Can you work these out from the model? Positions are in its coordinate system, mm. A direction names the side the tool comes from. Round coordinates to 2 decimals unless told otherwise and drop trailing zeros. Loops run counter-clockwise (first coordinate to the right, second up) from the corner with the lowest first, then second, coordinate; pieces in that order, holes last. Notation, with made-up numbers: M -23,-18 L 34,-18 A21 ccw 34,11 Z; hole C 70.25,20 d9. An arc over 180 degrees is marked long. Return JSON: item names as keys, results as strings.
```python
from build123d import *

# Parameters (mm, degrees)
CUT_EXTRUDE1_START     = -2.025
CUT_EXTRUDE1_OUTLINE_W = 3.186396103
CUT_EXTRUDE1_OUTLINE_H = 1.6
CUT_EXTRUDE1_DEPTH     = 4.05
CUT_EXTRUDE1_START_2   = -1.575
CUT_EXTRUDE1_2_DEPTH   = 1.425
CUT_EXTRUDE1_START_3   = 0.15
CUT_EXTRUDE1_3_DEPTH   = 1.425
SKETCH2_W              = 0.3
SKETCH2_H              = 3.186396103
CUT_EXTRUDE2_DEPTH     = 0.3
CUT_EXTRUDE3_DEPTH     = 0.186396103
SKETCH4_W              = 3.45
SKETCH4_H              = 3
CUT_EXTRUDE4_DEPTH     = 1
BOSS_EXTRUDE1_DEPTH    = 6.2
SKETCH6_W              = 2.55
SKETCH6_H              = 0.3
BOSS_EXTRUDE2_DEPTH    = 0.75
SKETCH7_W              = 0.3
SKETCH7_H              = 0.6
BOSS_EXTRUDE3_DEPTH    = 0.3
SKETCH8_W              = 0.3
SKETCH8_H              = 0.6
BOSS_EXTRUDE4_DEPTH    = 0.3
SKETCH9_W              = 3.15
SKETCH9_H              = 0.3
BOSS_EXTRUDE5_DEPTH    = 1
SKETCH10_W             = 0.3
SKETCH10_H             = 6.05
BOSS_EXTRUDE6_DEPTH    = 0.45
SKETCH11_W             = 1.5
SKETCH11_H             = 0.3
BOSS_EXTRUDE7_DEPTH    = 1.05
SKETCH12_W             = 1.5
SKETCH12_H             = 0.3
BOSS_EXTRUDE8_DEPTH    = 1
SKETCH13_W             = 0.3
SKETCH13_H             = 6.05
BOSS_EXTRUDE9_DEPTH    = 0.45
DRAFT1_ANGLE           = 45
DRAFT2_ANGLE           = 45
FILLET1_R              = 0.15
FILLET2_R              = 0.45
FILLET3_R              = 0.6


with BuildPart() as part:
    # Cut-Extrude1: read off the stored shape, not the designer's step
    # Cut-Extrude1 outline → Cut-Extrude1 (new body)
    with BuildSketch(Plane.YZ.offset(CUT_EXTRUDE1_START)):
        with Locations((3.343198051, 0.8)):
            Rectangle(CUT_EXTRUDE1_OUTLINE_W, CUT_EXTRUDE1_OUTLINE_H)
    extrude(amount=CUT_EXTRUDE1_DEPTH)

    # Cut-Extrude1 2 outline → Cut-Extrude1 2 (add)
    with BuildSketch(Plane.YZ.offset(CUT_EXTRUDE1_START_2)):
        Polygon((4.936396103, 1.6), (4.936396103, 1.3), (5.73137085, 2.094974747), (4.812132034, 3.014213562), (4.812132034, 1.6), align=None)
        Polygon((1.189495749, 1.3), (1.75, 1.3), (1.75, 1.6), (1.15, 1.6), (-1.128726234, 0.989417146), (-2.09465206, 1.248236191), (-2.172297774, 0.958458443), (-1.128726234, 0.678834292), align=None)
    extrude(amount=CUT_EXTRUDE1_2_DEPTH)

    # Cut-Extrude1 3 outline → Cut-Extrude1 3 (add)
    with BuildSketch(Plane.YZ.offset(CUT_EXTRUDE1_START_3)):
        Polygon((4.936396103, 1.6), (4.936396103, 1.3), (5.73137085, 2.094974747), (4.812132034, 3.014213562), (4.812132034, 1.6), align=None)
        Polygon((1.189495749, 1.3), (1.75, 1.3), (1.75, 1.6), (1.15, 1.6), (-1.128726234, 0.989417146), (-2.09465206, 1.248236191), (-2.172297774, 0.958458443), (-1.128726234, 0.678834292), align=None)
    extrude(amount=CUT_EXTRUDE1_3_DEPTH)

    # Sketch2 → Cut-Extrude2 (cut)
    with BuildSketch(Plane.XY.offset(1.6)):
        with Locations((0, 3.343198051)):
            Rectangle(SKETCH2_W, SKETCH2_H)
    extrude(amount=-CUT_EXTRUDE2_DEPTH, mode=Mode.SUBTRACT)

    # Sketch3 → Cut-Extrude3 (cut)
    with BuildSketch(Plane(origin=(0, 4.936396103, 0), x_dir=(-1, 0, 0), z_dir=(0, 1, 0))):
        Polygon((-1.575, 1.3), (-1.575, 1.6), (-2.025, 1.6), (-2.025, 0), (2.025, 0), (2.025, 1.6), (1.575, 1.6), (1.575, 1.3), (0.15, 1.3), (-0.15, 1.3), align=None)
    extrude(amount=-CUT_EXTRUDE3_DEPTH, mode=Mode.SUBTRACT)

    # Sketch4 → Cut-Extrude4 (cut)
    with BuildSketch(Plane.XY.offset(1.3)):
        with Locations((0, 3.25)):
            Rectangle(SKETCH4_W, SKETCH4_H)
    extrude(amount=-CUT_EXTRUDE4_DEPTH, mode=Mode.SUBTRACT)

    # Sketch5 → Boss-Extrude1 (add)
    with BuildSketch(Plane.XZ.offset(-1.75)):
        Polygon((-1.725, 0.85), (-1.725, 0.3), (1.725, 0.3), (1.725, 0.85), (2.025, 0.85), (2.025, 0), (-2.025, 0), (-2.025, 0.85), align=None)
    extrude(amount=BOSS_EXTRUDE1_DEPTH)

    # Sketch6 → Boss-Extrude2 (add)
    with BuildSketch(Plane(origin=(0, 4.75, 0), x_dir=(-1, 0, 0), z_dir=(0, 1, 0))):
        with Locations((0, 0.15)):
            Rectangle(SKETCH6_W, SKETCH6_H)
    extrude(amount=BOSS_EXTRUDE2_DEPTH)

    # Sketch7 → Boss-Extrude3 (add)
    with BuildSketch(Plane.ZY.offset(1.275)):
        with Locations((0.15, 5.2)):
            Rectangle(SKETCH7_W, SKETCH7_H)
    extrude(amount=BOSS_EXTRUDE3_DEPTH)

    # Sketch8 → Boss-Extrude4 (add)
    with BuildSketch(Plane(origin=(1.275, 0, 0), x_dir=(0, 0, -1), z_dir=(1, 0, 0))):
        with Locations((-0.15, 5.2)):
            Rectangle(SKETCH8_W, SKETCH8_H)
    extrude(amount=BOSS_EXTRUDE4_DEPTH)

    # Sketch9 → Boss-Extrude5 (add)
    with BuildSketch(Plane(origin=(0, 0, 0), x_dir=(-1, 0, 0), z_dir=(0, 0, -1))):
        with Locations((0, 5.35)):
            Rectangle(SKETCH9_W, SKETCH9_H)
    extrude(amount=BOSS_EXTRUDE5_DEPTH)

    # Sketch10 → Boss-Extrude6 (add)
    with BuildSketch(Plane.XY.offset(0.85)):
        with Locations((-1.875, -1.425)):
            Rectangle(SKETCH10_W, SKETCH10_H)
    extrude(amount=BOSS_EXTRUDE6_DEPTH)

    # Sketch11 → Boss-Extrude7 (add)
    with BuildSketch(Plane.XZ.offset(4.45)):
        with Locations((0, 0.15)):
            Rectangle(SKETCH11_W, SKETCH11_H)
    extrude(amount=BOSS_EXTRUDE7_DEPTH)

    # Sketch12 → Boss-Extrude8 (add)
    with BuildSketch(Plane(origin=(0, 0, 0), x_dir=(-1, 0, 0), z_dir=(0, 0, -1))):
        with Locations((0, -5.35)):
            Rectangle(SKETCH12_W, SKETCH12_H)
    extrude(amount=BOSS_EXTRUDE8_DEPTH)

    # Sketch13 → Boss-Extrude9 (add)
    with BuildSketch(Plane.XY.offset(0.85)):
        with Locations((1.875, -1.425)):
            Rectangle(SKETCH13_W, SKETCH13_H)
    extrude(amount=BOSS_EXTRUDE9_DEPTH)

    # Draft1
    draft1_faces = [part.faces().sort_by_distance(p)[0] for p in [
        (0.8625, 4.812132034, 2.307106781),
    ]]
    draft(draft1_faces, Plane(origin=(0.960282071, 3.25, 1.6), x_dir=(1, 0, 0), z_dir=(0, 0, 1)), DRAFT1_ANGLE)

    # Draft2
    draft2_faces = [part.faces().sort_by_distance(p)[0] for p in [
        (-0.8625, 4.812132034, 2.307106781),
    ]]
    draft(draft2_faces, Plane(origin=(0.960282071, 3.25, 1.6), x_dir=(1, 0, 0), z_dir=(0, 0, 1)), DRAFT2_ANGLE)

    # Fillet1
    fillet1_edges = [part.edges().sort_by_distance(p)[0] for p in [
        (1.725, 3.25, 1.3),
        (0.8625, 1.189495749, 1.3),
        (0, -5.2, 0),
        (-0.8625, 4.812132034, 1.6),
        (0, 5.2, 0),
        (-1.725, 0.15, 0.3),
        (-0.8625, -1.128726234, 0.989417146),
        (-1.725, 3.25, 1.3),
        (0.8625, 4.812132034, 1.6),
        (0.8625, -1.128726234, 0.989417146),
        (-0.8625, 1.189495749, 1.3),
        (1.725, 0.15, 0.3),
    ]]
    fillet(fillet1_edges, radius=FILLET1_R)

    # Fillet2
    fillet2_edges = [part.edges().sort_by_distance(p)[0] for p in [
        (-2.025, 3.25, 1.6),
        (1.575, -2.133474917, 1.103347317),
        (0.15, -2.133474917, 1.103347317),
        (0.8625, -1.128726234, 0.678834292),
        (-0.8625, 4.936396103, 1.3),
        (0, 5.5, 0.3),
        (-0.8625, 1.15, 1.6),
        (2.025, 3.25, 1.6),
        (-0.15, -2.133474917, 1.103347317),
        (-1.575, -2.133474917, 1.103347317),
        (2.025, 0.15, 0),
        (-2.025, 0.15, 0),
        (0, -5.5, 0.3),
        (-0.8625, -1.128726234, 0.678834292),
        (0.8625, 4.936396103, 1.3),
        (0.8625, 1.15, 1.6),
    ]]
    fillet(fillet2_edges, radius=FILLET2_R)

    # Fillet3
    fillet3_edges = [part.edges().sort_by_distance(p)[0] for p in [
        (1.575, 5.625304833, 2.201040764),
        (1.875, -4.45, 1.3),
        (-1.875, -4.45, 1.3),
        (-0.75, -4.45, 0.15),
        (-1.575, 5.625304833, 2.201040764),
        (0.75, -4.45, 0.15),
    ]]
    fillet(fillet3_edges, radius=FILLET3_R)


solid = part.part
```
Q1. Thinking about a two-plate mould opening in X: for faces 1 (the flat face through (-2.025, 0, 1)), 2 (the flat face through (-1.725, 0, 1)), 3 (the flat face through (1, 3, 1.6)), which applies, pulls with the +X half, pulls with the -X half, needs draft (parallel to the pull), parting line crosses it, or undercut?
Results:
{"face 1": "pulls with the -X half", "face 2": "undercut", "face 3": "needs draft"}
Q2. Suppose I cut it at C-C, the plane z = 0.15. Please give me the cut outline in (x, y) (3 decimals), plus the area to 3 significant figures.
Results:
{"outline": "M -1.91,-4.45 L -1.35,-4.45 A0.6 cw -0.75,-5.05 L -0.75,-5.385 L 0.75,-5.385 L 0.75,-5.05 A0.6 cw 1.35,-4.45 L 1.91,-4.45 L 1.91,4.75 L 1.275,4.75 L 1.275,4.9 L 1.575,4.9 L 1.575,5.385 L -1.575,5.385 L -1.575,4.9 L -1.275,4.9 L -1.275,4.75 L -1.91,4.75 Z", "area": "38.6 mm2"}
Q3. Suppose I cut it at D-D, the plane y = 2.25. Please give me the cut outline in (x, z) (3 decimals), plus the area to 3 significant figures.
Results:
{"outline": "M -2.025,0.45 A0.45 ccw -1.575,0 L 1.575,0 A0.45 ccw 2.025,0.45 L 2.025,1.15 A0.45 ccw 1.575,1.6 L 0.15,1.6 L 0.15,1.3 L 1.575,1.3 A0.15 cw 1.725,1.15 L 1.725,0.45 A0.15 cw 1.575,0.3 L -1.575,0.3 A0.15 cw -1.725,0.45 L -1.725,1.15 A0.15 cw -1.575,1.3 L -0.15,1.3 L -0.15,1.6 L -1.575,1.6 A0.45 ccw -2.025,1.15 Z", "area": "2.79 mm2"}
Q4. Suppose I cut it at A-A, the plane y = -2.75. Please give me the cut outline in (x, z) (3 decimals).
Results:
{"outline": "M -2.025,0.45 A0.45 ccw -1.575,0 L 1.575,0 A0.45 ccw 2.025,0.45 L 2.025,1.3 L 1.725,1.3 L 1.725,0.45 A0.15 cw 1.575,0.3 L -1.575,0.3 A0.15 cw -1.725,0.45 L -1.725,1.3 L -2.025,1.3 Z"}
Q5. I'm going to push flat-ended pins straight in: pin 1 Ø1.6 at (x, y) = (1, 3.5) entering from -Z; pin 2 Ø1.5 at (x, z) = (0.5, 0) entering from +Y; pin 3 Ø0.5 at (x, z) = (-1.5, 0.5) entering from -Y. Where does each tip first touch, or does it pass through?
Results:
{"pin 1": "stops at z = 0", "pin 2": "stops at y = 5.5", "pin 3": "stops at y = -4.45"}
Q6. If I drill on line 1 along Z through (x, y) = (-0.4, 4); line 2 along X through (y, z) = (-3.5, 0.85) (3 decimals); line 3 along Y through (x, z) = (-0.2, -0.65), over which ranges is the centre line in solid material (lowest first)?
Results:
{"line 1": "z = 0 to 0.3, 1.3 to 1.6", "line 2": "x = -2.025 to -1.725, 1.725 to 2.025", "line 3": "y = -5.5 to -5.2, 5.2 to 5.5"}
Q7. On a 3-axis mill with a long thin cutter (end or side, diameter ignored), from which of +Z, -Z, +X, -X, +Y, -Y can I reach the whole of each face in a straight line? I mean faces 4 (the flat face through (0.853, -1.715, 0.836)), 5 (the flat face through (0, 0, 0.3)), 6 (the flat face through (-0.87, -1.62, 1.12)), 7 (the flat face through (1, 3, 1.3)). Say none if no direction works.
Results:
{"face 4": "-Y", "face 5": "+Y, -Y", "face 6": "+Z", "face 7": "+Y"}
